Autodesk Inventor part; units mm, degrees
ref_plane "作業平面1" through (0, 0, 9.6) normal (0, 0, 1) x (1, 0, 0)
ref_plane "作業平面2" through (-9.9, 0, 36) normal (0, 1, 0) x (1, 0, 0)
ref_plane "作業平面3" through (0, 0, 8.35) normal (0, 0, -1) x (-1, 0, 0)
sketch "スケッチ1" plane through (0, 0, 0) normal (0, 0, 1) x (1, 0, 0)
  line L0 (9.9, -20.2) -> (-9.9, -20.2)
  line L1 (-9.9, -20.2) -> (-9.9, 20.2)
  line L2 (-9.9, 20.2) -> (9.9, 20.2)
  line L3 (9.9, 20.2) -> (9.9, -20.2)
  line L4 (9.9, -20.2) -> (-9.9, 20.2) construction
  line L5 (-9.9, -20.2) -> (9.9, 20.2) construction
  circle A0 centre (-10.932, 25.3443) radius 2.25
  point P0 (0, 0)
  dimension "d0" = 4.5
  dimension "d1" = 40.4
  dimension "d2" = 19.8
extrude "押し出し1" add sketch "スケッチ1" along normal blind 36 contours L0 L1 L2 L3
sketch "スケッチ2" plane through (0, 0, 0) normal (0, 0, -1) x (-1, 0, 0)
  circle A0 centre (0, 10.2) radius 3
  line L0 (9.9, 20.2) -> (-9.9, 20.2)
  point P0 (0, 0)
  dimension "d5" = 6
  dimension "d6" = 10
extrude "押し出し2" add sketch "スケッチ2" along normal blind 6.2
ref_plane "作業平面1" through (0, 0, 9.6) normal (0, 0, 1) x (1, 0, 0)
sketch "スケッチ4" plane through (0, 0, 9.6) normal (0, 0, 1) x (1, 0, 0)
  line L0 (-9.9, -20.2) -> (9.9, -20.2)
  line L1 (9.9, -20.2) -> (9.9, 20.2)
  line L2 (9.9, 20.2) -> (-9.9, 20.2)
  line L3 (-9.9, 20.2) -> (-9.9, -20.2)
  line L4 (-9.9, 20.2) -> (9.9, 20.2)
  line L5 (9.9, 20.2) -> (9.9, 27.7)
  line L6 (9.9, 27.7) -> (-9.9, 27.7)
  line L7 (-9.9, 27.7) -> (-9.9, 20.2)
  line L8 (-9.9, -20.2) -> (9.9, -20.2)
  line L9 (9.9, -20.2) -> (9.9, -27.7)
  line L10 (9.9, -27.7) -> (-9.9, -27.7)
  line L11 (-9.9, -27.7) -> (-9.9, -20.2)
  circle A0 centre (-5, 24.4) radius 1.5
  circle A1 centre (5, 24.4) radius 1.5
  line L12 (0, 27.7) -> (0, 20.2)
  point P0 (0, 0)
  dimension "d10" = 7.5
  dimension "d11" = 7.5
  dimension "d12" = 3
  dimension "d13" = 4.2
  dimension "d15" = 10
  dimension "d16" = 5
  dimension "d17" = 4.2
extrude "押し出し3" add sketch "スケッチ4" against normal blind 2.5 contours L7 L6 L12 L2 | L2 L12 L6 L5
ref_plane "作業平面2" through (-9.9, 0, 36) normal (0, 1, 0) x (1, 0, 0)
mirror "ミラー1" about plane through (-9.9, 0, 36) normal (0, 1, 0) of "押し出し3"
sketch "スケッチ5" plane through (0, 0, 7.1) normal (0, 0, -1) x (-1, 0, 0)
  circle A0 centre (5, 24.4) radius 1.5
  circle A1 centre (-5, 24.4) radius 1.5
  line L0 (9.9, 20.2) -> (-9.9, 20.2)
  line L1 (9.9, 20.2) -> (9.9, 27.7)
  line L2 (9.9, 27.7) -> (-9.9, 27.7)
  line L3 (-9.9, 27.7) -> (-9.9, 20.2)
  circle A2 centre (5, -24.4) radius 1.5
  circle A3 centre (-5, -24.4) radius 1.5
  line L4 (-9.9, -20.2) -> (9.9, -20.2)
  line L5 (-9.9, -27.7) -> (-9.9, -20.2)
  line L6 (9.9, -27.7) -> (-9.9, -27.7)
  line L7 (9.9, -20.2) -> (9.9, -27.7)
  circle A4 centre (-5, 24.4) radius 4
  circle A5 centre (5, 24.4) radius 4
  circle A6 centre (-5, -24.4) radius 4
  circle A7 centre (5, -24.4) radius 4
  point P0 (0, 0)
  dimension "d20" = 8
  dimension "d21" = 8
  dimension "d22" = 8
  dimension "d23" = 8
extrude "押し出し4" add sketch "スケッチ5" along normal blind 1.5 contours A5 L2 | L2 A5 | A4 L2 | L2 A4 | A6 L6 | L6 A6 | A7 L6 | L6 A7
ref_plane "作業平面3" through (0, 0, 8.35) normal (0, 0, -1) x (-1, 0, 0)
mirror "ミラー2" about plane through (0, 0, 8.35) normal (0, 0, -1) of "押し出し4"
ref_plane "作業平面4" through (0, -20.2, 0) normal (-1, 0, 0) x (0, 0, 1)
equation "\"d16\" = 0.5 * d15"
equation "\"d17\" = d13"
Geometry: final body of the model. Coordinates: model frame, mm. A direction names the side the tool comes from. Round coordinates to 2 decimals unless told otherwise and drop trailing zeros. Order: outer loops, then holes, each group sorted by start corner. A loop starts at its lowest first (then second) coordinate and runs counter-clockwise, first axis right, second up.
Q1. Section C-C, the plane y = 10.2. Output: boundary loops of the cut face in (x, z).
Result sheet:
outline: (-9.9, 0) - (-3, 0) - (-3, -6.2) - (3, -6.2) - (3, 0) - (9.9, 0) - (9.9, 36) - (-9.9, 36) - close
Q2. Section B-B, the plane y = 24.4. Output: boundary loops of the cut face in (x, z).
Result sheet:
outline: (-9.9, 7.1) - (-9, 7.1) - (-9, 5.6) - (-6.5, 5.6) - (-6.5, 11.1) - (-9, 11.1) - (-9, 9.6) - (-9.9, 9.6) - close; (-3.5, 5.6) - (-1, 5.6) - (-1, 7.1) - (1, 7.1) - (1, 5.6) - (3.5, 5.6) - (3.5, 11.1) - (1, 11.1) - (1, 9.6) - (-1, 9.6) - (-1, 11.1) - (-3.5, 11.1) - close; (6.5, 5.6) - (9, 5.6) - (9, 7.1) - (9.9, 7.1) - (9.9, 9.6) - (9, 9.6) - (9, 11.1) - (6.5, 11.1) - close
Q3. Material intervals for probe 1 along X at (y, z) = (-24.4, 6.85); probe 2 along Y at (x, z) = (5, 6.2); probe 3 along X at (y, z) = (24.4, 8.75), sorted ascending.
Result sheet:
probe 1: x = -9 to -6.5, -3.5 to -1, 1 to 3.5, 6.5 to 9
probe 2: y = -28.4 to -25.9, -22.9 to -20.4, -20.2 to 20.2, 20.4 to 22.9, 25.9 to 28.4
probe 3: x = -9.9 to -6.5, -3.5 to 3.5, 6.5 to 9.9
Q4. Pin query (flat end, axial travel): pin 1 (0.8 mm diameter, centred on x = 4, y = 28, fed in from -Z); pin 2 (2.5 mm diameter, centred on x = 5, y = 24.4, fed in from +Z); pin 3 (10 mm diameter, centred on x = 0.5, z = 17.5, fed in from +Y); pin 4 (2 mm diameter, centred on x = 1, y = -0.5, fed in from -Z). Return the tip coordinate at first contact, or that it passes through.
Result sheet:
pin 1: stops at z = 5.6
pin 2: passes through
pin 3: stops at y = 20.2
pin 4: stops at z = 0
Q5. Access query for faces 1 (the face through (0, -20.2, 4)), 2 (the face through (5.1, 22.7, 5.6)), 3 (the face through (-4.9, -26.1, 5.6)), 4 (the face through (-5.1, -26.1, 11.1)), 5 (the face through (5.867, 20.495, 10.34)). Directions: +Z, -Z, +X, -X, +Y, -Y. A direction counts if a zero-diameter tool reaches every point of the face in a straight line with its end or side. Return the directions, or none.
Result sheet:
face 1: -Z, +X, -X
face 2: -Z, +X, -X, +Y
face 3: -Z, +X, -X, -Y
face 4: +Z, +X, -X, -Y
face 5: +Z
Q6. Section D-D, the plane z = 26.5. Output: boundary loops of the cut face in (x, y), and give its area (3 significant figures).
Result sheet:
outline: (-9.9, -20.2) - (9.9, -20.2) - (9.9, 20.2) - (-9.9, 20.2) - close
area: 800 mm2
